```python
from build123d import *

# Parameters (mm, degrees)
F1_DEPTH = 254


with BuildPart() as f1:
    # F0 (on Right) → F1 (new body)
    with BuildSketch(Plane.YZ):
        Polygon((72.399652, -4.747743), (71.772374, -4.579188), (69.902299, -4.091153), (66.821634, -3.323184), (62.581714, -2.320747), (57.257264, -1.120419), (50.93622, 0.235229), (43.729961, 1.692021), (35.760152, 3.183992), (27.163039, 4.63931), (18.086705, 5.978855), (8.685022, 7.130796), (-0.879348, 8.030667), (-10.443743, 8.630082), (-19.845426, 8.899754), (-24.434165, 8.908542), (-28.921761, 8.832317), (-33.289189, 8.674049), (-37.518848, 8.43661), (-41.591713, 8.111261), (-45.488682, 7.68477), (-49.195126, 7.142505), (-52.694942, 6.4786), (-55.973447, 5.70771), (-59.015986, 4.854753), (-61.807928, 3.956355), (-64.340435, 3.038881), (-66.601823, 2.106778), (-68.580356, 1.154151), (-70.270167, 0.164897), (-71.66102, -0.861009), (-72.749943, -1.900123), (-73.531095, -2.9099), (-74.001554, -3.84495), (-74.158348, -4.678858), (-74.001554, -5.411648), (-73.531095, -6.063818), (-72.749943, -6.647129), (-71.66102, -7.167397), (-70.270167, -7.618806), (-68.580356, -7.992542), (-66.601823, -8.285658), (-64.340435, -8.509889), (-61.807928, -8.675497), (-59.015986, -8.797138), (-55.973447, -8.874811), (-52.694942, -8.908517), (-49.195126, -8.898255), (-45.488682, -8.844026), (-41.591713, -8.754643), (-37.518848, -8.635924), (-33.289189, -8.498154), (-28.921761, -8.350123), (-24.434165, -8.193303), (-19.845426, -8.033563), (-10.443743, -7.705268), (-0.879348, -7.374052), (8.685022, -7.042836), (18.086705, -6.718935), (27.163039, -6.405296), (35.760152, -6.107786), (43.729961, -5.83372), (50.93622, -5.590438), (57.257264, -5.376469), (62.581714, -5.190338), (66.821634, -5.026203), (69.902299, -4.885512), (71.772374, -4.784369), align=None)
    extrude(amount=F1_DEPTH)


solid = f1.part
```
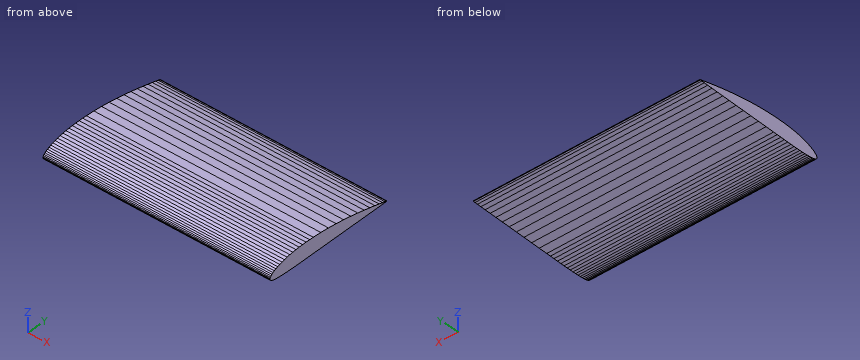
Input: part model. Units: mm. Frame: model coordinates. Round coordinates to 2 decimals unless told otherwise and drop trailing zeros. Loops run counter-clockwise (first coordinate to the right, second up) from the corner with the lowest first, then second, coordinate; pieces in that order, holes last. Notation, with made-up numbers: (57, 54.5) -> (75, 54.5) arc R15 cw to (75, 74.5) -> close; hole circle Ø6 at (-10.75, -13). An arc over 180 degrees is marked (long way). Write each question's results on one line, items separated by ' | '.
1. Ray query, line 1 (Z direction, x = 178.5, y = 27.5); line 2 (Z direction, x = 80.5, y = -59.5). Return the intervals inside material, ascending. Write a range as from..to.
Geometry results:
line 1: -6.39..4.58 | line 2: -8.78..4.7
2. First-contact query: P1, Ø1.5, axis at x = 42, z = 3.5, coming from the -Y side; P2, Ø10, axis at x = 29, y = -20, coming from the +Z side; P3, Ø5, axis at x = 78.5, y = 45, coming from the +Z side; P4, Ø10, axis at x = 151, z = -5, coming from the -Y side. Flat tips, straight axial feed; report the tip coordinate or a pass-through.
Geometry results:
P1: y = -65.04 | P2: z = 8.91 | P3: z = 1.92 | P4: y = -74.16
3. Section A-A (y = 22.5). Return loops of the section in (x, z).
Geometry results:
outline: (0, -6.57) -> (254, -6.57) -> (254, 5.33) -> (0, 5.33) -> close
